Drawing for the job (mm, zero at the part's lowest x, y, z). A direction names the side the tool comes from. Round coordinates to 2 decimals unless told otherwise and drop trailing zeros. Order: outer loops, then holes, each group sorted by start corner. A loop starts at its lowest first (then second) coordinate and runs counter-clockwise, first axis right, second up. Notation, with made-up numbers: (-11, 45.25) -> (7, 45.25) arc R21 ccw to (7, 84.25) -> close; hole circle Ø11 at (-38, 24.25). An arc over 180 degrees is marked (long way). Use CSV: the item, a comma, the result in double quotes.
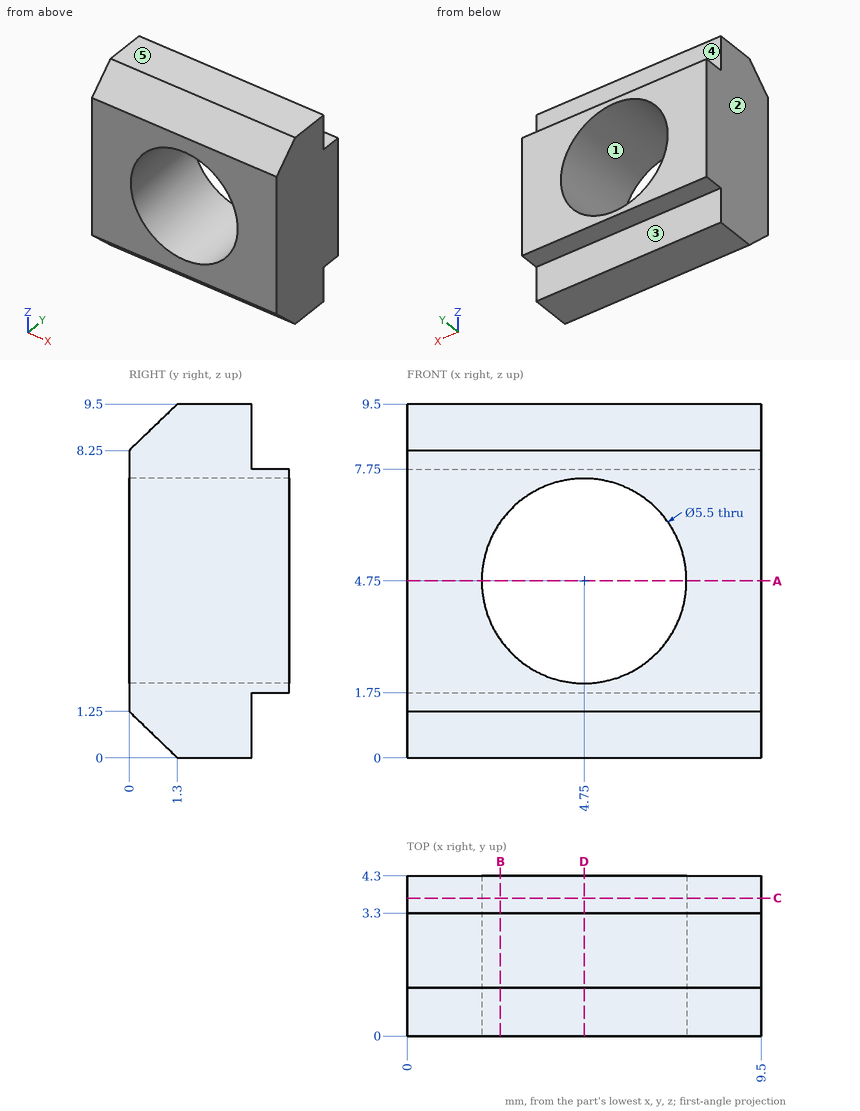
Q1. Which spindle directions (+Z, -Z, +X, -X, +Y, -Y) get a long thin tool onto all of the face, cutting with end or side? Do the marked faces 4 and 5. Say none if no direction does.
From the geometry:
face 4,"+Z, +X, -X, +Y"
face 5,"+Z, +X, -X, +Y, -Y"
Q2. Mould opens along X. For the marked faces 1, 2 and 3 say: +X half, -X half, draft (parallel to the pull), parting line (faces both ways), or undercut.
From the geometry:
face 1,"undercut"
face 2,"-X half"
face 3,"draft"
Q3. Cut at B-B (x = 2.5). Give the cut face in (y, z).
From the geometry:
outline,"(0, 1.25) -> (1.3, 0) -> (3.3, 0) -> (3.3, 1.75) -> (4.3, 1.75) -> (4.3, 3.17) -> (0, 3.17) -> close; (0, 6.33) -> (4.3, 6.33) -> (4.3, 7.75) -> (3.3, 7.75) -> (3.3, 9.5) -> (1.3, 9.5) -> (0, 8.25) -> close"
Q4. Cut at D-D (x = 4.75). Give the cut face in (y, z).
From the geometry:
outline,"(0, 1.25) -> (1.3, 0) -> (3.3, 0) -> (3.3, 1.75) -> (4.3, 1.75) -> (4.3, 2) -> (0, 2) -> close; (0, 7.5) -> (4.3, 7.5) -> (4.3, 7.75) -> (3.3, 7.75) -> (3.3, 9.5) -> (1.3, 9.5) -> (0, 8.25) -> close"
Q5. Pin check, flat tips, straight feed: pin 1 (0.5 mm diameter, centred on x = 3.5, y = 4, fed in from -Z); pin 2 (0.8 mm diameter, centred on x = 5, y = 4, fed in from +Z); pin 3 (0.9 mm diameter, centred on x = 7, z = 9, fed in from +Y). Stop position of each tip, or through.
From the geometry:
pin 1,"stops at z = 1.75"
pin 2,"stops at z = 7.75"
pin 3,"stops at y = 3.3"
Q6. Cut at C-C (y = 3.7). Give the cut face in (x, z).
From the geometry:
outline,"(0, 1.75) -> (9.5, 1.75) -> (9.5, 7.75) -> (0, 7.75) -> close; hole circle Ø5.5 at (4.75, 4.75)"
Q7. Cut at A-A (z = 4.75). Give the cut face in (x, y).
From the geometry:
outline,"(0, 0) -> (2, 0) -> (2, 4.3) -> (0, 4.3) -> close; (7.5, 0) -> (9.5, 0) -> (9.5, 4.3) -> (7.5, 4.3) -> close"
Q8. Probe line 1 along Z through (x, y) = (4.75, 1.5); line 2 along X through (y, z) = (2.1, 2.5); line 3 along Y through (x, z) = (7.25, 8). List the from-to ranges inside material, lowest first.
From the geometry:
line 1,"z = 0 to 2, 7.5 to 9.5"
line 2,"x = 0 to 3.17, 6.33 to 9.5"
line 3,"y = 0 to 3.3"
